For this review, use the dimensioned drawing (mm, ordinates from the lowest corner) and the shaded views. A direction names the side the tool comes from. Round coordinates to 2 decimals unless told otherwise and drop trailing zeros. Loops run counter-clockwise (first coordinate to the right, second up) from the corner with the lowest first, then second, coordinate; pieces in that order, holes last. Notation, with made-up numbers: M 16.5,-18.75 L 74.5,-18.75 A20 cw 74.5,1.25 Z; hole C -12,15.5 d5. An arc over 180 degrees is marked long. Answer as a JSON object with one key per item and string values. Group by question number.
Item 1: The part is to be moulded in two halves that separate along X. For the marked faces 1, 2 and 3, say which applies: +X half, -X half, draft (parallel to the pull), parting line (faces both ways), or undercut.
Item 2: Insertion check: P1, Ø10, axis at x = 17, y = 4.5, coming from the -Z side; P2, Ø12.5, axis at y = 16, z = 27, coming from the +X side; P3, Ø1.5, axis at x = 3.5, y = 22.5, coming from the +Z side; P4, Ø6, axis at x = 50, z = 15, coming from the +Y side. Each pin has a flat end and moves straight along its axis. Give the tip position at first contact, or say it passes through.
Item 3: Tool access review of the marked faces 4, 5 and 6: name each direction out of +Z, -Z, +X, -X, +Y, -Y from which nothing blocks a thin tool from reaching the whole face with its end or side.
Item 4: Consider section C-C (y = 24). Give the boundary of the cut face in (x, z).
Item 5: Consider section A-A (z = 15). Give the boundary of the cut face in (x, y), and give its area (3 significant figures).
Item 6: Consider section B-B (x = 50). Give the boundary of the cut face in (y, z), and give its area (3 significant figures).
Item 7: To check wall thickness, follow line 1 (Y direction, x = 25, z = 25.5); line 2 (X direction, y = 15.5, z = 13.5); line 3 (Z direction, x = 24, y = 12.5). State the ranges of each line that lie inside material, in increasing order.
Item 8: Consider section D-D (x = 7). Give the boundary of the cut face in (y, z).
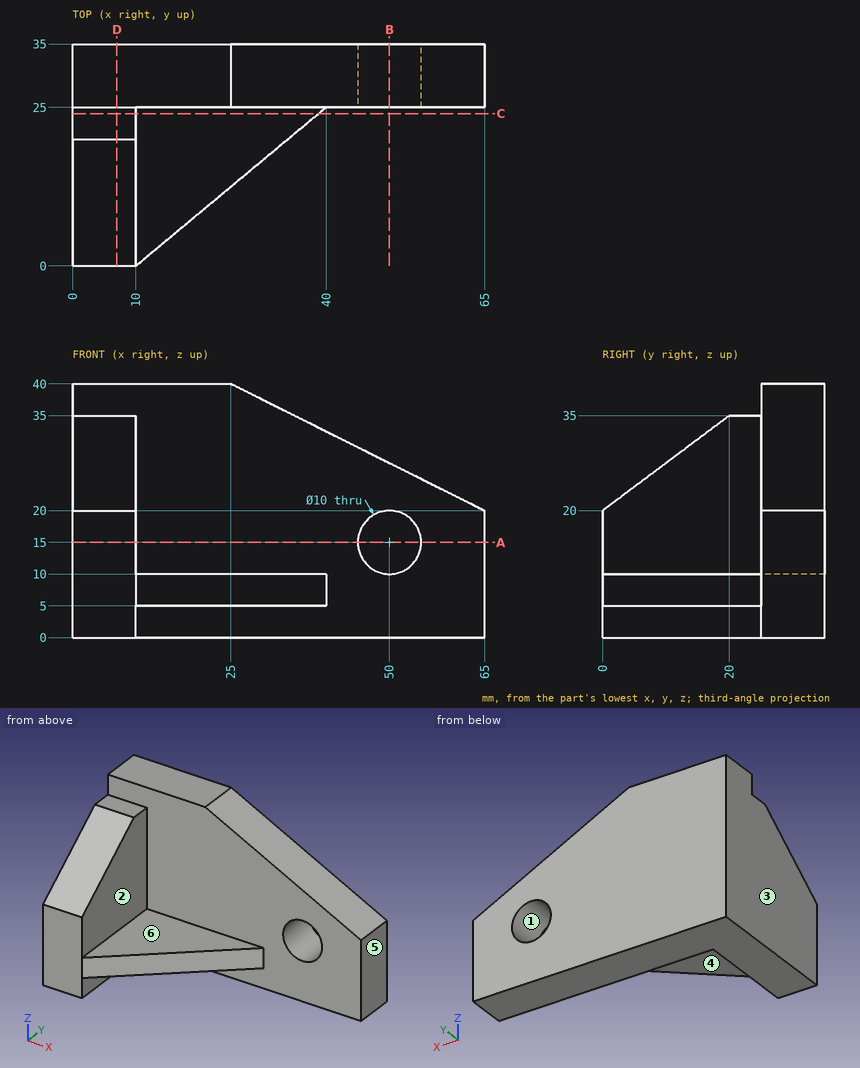
Geometry results:
{
 "1": {"face 1": "undercut", "face 2": "+X half", "face 3": "-X half"},
 "2": {"P1": "stops at z = 5", "P2": "stops at x = 10", "P3": "stops at z = 35", "P4": "passes through"},
 "3": {"face 4": "-Z, +X, -Y", "face 5": "+Z, -Z, +X, +Y, -Y", "face 6": "+Z, +X, -Y"},
 "4": {"outline": "M 0,0 L 10,0 L 10,5 L 38.8,5 L 38.8,10 L 10,10 L 10,35 L 0,35 Z"},
 "5": {"outline": "M 0,0 L 10,0 L 10,25 L 45,25 L 45,35 L 0,35 Z; M 55,25 L 65,25 L 65,35 L 55,35 Z", "area": "800 mm^2"},
 "6": {"outline": "M 25,0 L 35,0 L 35,10 L 25,10 Z; M 25,20 L 35,20 L 35,27.5 L 25,27.5 Z", "area": "175 mm^2"},
 "7": {"line 1": "y = 25 to 35", "line 2": "x = 0 to 10", "line 3": "z = 5 to 10"},
 "8": {"outline": "M 0,0 L 35,0 L 35,40 L 25,40 L 25,35 L 20,35 L 0,20 Z"}
}
